```python
from build123d import *
from build123d.topology import SkipClean

# Parameters (mm, degrees)
EXTRUDE_1_DEPTH       = 200
MIRROR_2_COPY_1_DEPTH = 200
FILLET_1_R            = 2


with BuildPart() as part:
    # Sketch 1 → Extrude 1 (new, symmetric)
    with BuildSketch(Plane.XY):
        with BuildLine():
            Line((3, 14), (0, 14))
            Line((0, 14), (0, 12.5))
            ThreePointArc((0, 12.5), (1.767766953, 11.767766953), (2.5, 10))
            ThreePointArc((2.5, 10), (1.767766953, 8.232233047), (0, 7.5))
            Line((0, 7.5), (0, 6))
            Line((0, 6), (3, 6))
            Line((3, 6), (5.5, 3.5))
            Line((5.5, 3.5), (5.991970664, 3))
            Line((5.991970664, 3), (8, 3))
            Line((8, 3), (8, 0))
            Line((8, 0), (10, 0))
            Line((10, 0), (10, 5.641940268))
            ThreePointArc((10, 5.641940268), (9.646446609, 5.788386877), (9.5, 6.141940268))
            Line((9.5, 6.141940268), (8, 6.141940268))
            Line((8, 6.141940268), (8, 4.641940268))
            Line((8, 4.641940268), (6.5, 4.641940268))
            Line((6.5, 4.641940268), (4.740462433, 6.401477835))
            Line((4.740462433, 6.401477835), (4.740462433, 13.598522165))
            Line((4.740462433, 13.598522165), (6.5, 15.358059732))
            Line((6.5, 15.358059732), (8, 15.358059732))
            Line((8, 15.358059732), (8, 13.858059732))
            Line((8, 13.858059732), (9.5, 13.858059732))
            ThreePointArc((9.5, 13.858059732), (9.646446609, 14.211613123), (10, 14.358059732))
            Line((10, 14.358059732), (10, 20))
            Line((10, 20), (4.5, 20))
            ThreePointArc((4.5, 20), (4.353553391, 19.646446609), (4, 19.5))
            Line((4, 19.5), (4, 18))
            Line((4, 18), (5.5, 18))
            Line((5.5, 18), (5.5, 16.5))
            Line((5.5, 16.5), (3, 14))
        make_face()
    extrude_1 = extrude(amount=EXTRUDE_1_DEPTH, both=True)

    # Mirror 1: Extrude 1 across plane
    with SkipClean():  # the faces are left unmerged after this step: merging them gives an invalid solid
        add(extrude_1.mirror(Plane(origin=(0, 0, 0), x_dir=(0, 0, 1), z_dir=(1, 0, 0))))

    # Mirror 2: Extrude 1 across plane
    with SkipClean():  # the faces are left unmerged after this step: merging them gives an invalid solid
        add(extrude_1.mirror(Plane.ZX))

    # Mirror 2 copy 1 sketch → Mirror 2 copy 1 (add, symmetric)
    with SkipClean():  # the faces are left unmerged after this step: merging them gives an invalid solid
        with BuildSketch(Plane(origin=(0, 0, 0), x_dir=(-1, 0, 0), z_dir=(0, 0, 1))):
            with BuildLine():
                Line((3, 14), (0, 14))
                Line((0, 14), (0, 12.5))
                ThreePointArc((0, 12.5), (1.767766953, 11.767766953), (2.5, 10))
                ThreePointArc((2.5, 10), (1.767766953, 8.232233047), (0, 7.5))
                Line((0, 7.5), (0, 6))
                Line((0, 6), (3, 6))
                Line((3, 6), (5.5, 3.5))
                Line((5.5, 3.5), (5.991970664, 3))
                Line((5.991970664, 3), (8, 3))
                Line((8, 3), (8, 0))
                Line((8, 0), (10, 0))
                Line((10, 0), (10, 5.641940268))
                ThreePointArc((10, 5.641940268), (9.646446609, 5.788386877), (9.5, 6.141940268))
                Line((9.5, 6.141940268), (8, 6.141940268))
                Line((8, 6.141940268), (8, 4.641940268))
                Line((8, 4.641940268), (6.5, 4.641940268))
                Line((6.5, 4.641940268), (4.740462433, 6.401477835))
                Line((4.740462433, 6.401477835), (4.740462433, 13.598522165))
                Line((4.740462433, 13.598522165), (6.5, 15.358059732))
                Line((6.5, 15.358059732), (8, 15.358059732))
                Line((8, 15.358059732), (8, 13.858059732))
                Line((8, 13.858059732), (9.5, 13.858059732))
                ThreePointArc((9.5, 13.858059732), (9.646446609, 14.211613123), (10, 14.358059732))
                Line((10, 14.358059732), (10, 20))
                Line((10, 20), (4.5, 20))
                ThreePointArc((4.5, 20), (4.353553391, 19.646446609), (4, 19.5))
                Line((4, 19.5), (4, 18))
                Line((4, 18), (5.5, 18))
                Line((5.5, 18), (5.5, 16.5))
                Line((5.5, 16.5), (3, 14))
            make_face()
        extrude(amount=MIRROR_2_COPY_1_DEPTH, both=True)

    # Fillet 1
    fillet_1_edges = [part.edges().sort_by_distance(p)[0] for p in [
        (-10, 20, 0),
        (-10, -20, 0),
        (10, -20, 0),
        (10, 20, 0),
    ]]
    fillet(fillet_1_edges, radius=FILLET_1_R)


solid = part.part
```
Build history of the part. All positions in model axes, mm. A direction names the side the tool comes from. Round coordinates to 2 decimals unless told otherwise and drop trailing zeros. Put each result on its own line as item: value.
Item 1: Flat gauge pins, fed straight in: P1, Ø1.5, axis at x = 5, y = -1.5, coming from the +Z side; P2, Ø6, axis at y = 9.5, z = -58.5, coming from the -X side; P3, Ø1.5, axis at y = -10.5, z = 58, coming from the +X side; P4, Ø0.8, axis at x = 8.5, z = -40.5, coming from the -Y side. Where does each tip first touch, or does it go through?
Here are the results:
P1: passes through
P2: stops at x = -4.74
P3: stops at x = 4.74
P4: stops at y = -20
Item 2: Wall check: probe 1 along Y at (x, z) = (-8.5, 37); probe 2 along Y at (x, z) = (-7.75, -19); probe 3 along X at (y, z) = (1.5, 107). Give the ranges that are in metal, low to high. Write a range as from..to.
Here are the results:
probe 1: y = -19.94..-13.86, -6.14..6.14, 13.86..19.94
probe 2: y = -20..-15.36, -4.64..-3, 3..4.64, 15.36..20
probe 3: x = -10..-8, 8..10
Item 3: Tool access for faces 3 (the face through (4.74, -10, 3)), 4 (the face through (-4.74, 10, 3)), 5 (the face through (5, -5, -200)): list every direction of +Z, -Z, +X, -X, +Y, -Y with a clear straight run to the whole face (end or side of a thin tool).
Here are the results:
face 3: +Z, -Z, +X
face 4: +Z, -Z, -X
face 5: -Z, +X, -X, +Y, -Y
Item 4: Two-plate mould, pull along Y, no slides. Class faces 1 (the face through (5, -5, 200)), 2 (the face through (-4.74, -10, 3)): pulls with the +Y half, pulls with the -Y half, needs draft (parallel to the pull), parting line crosses it, or undercut.
Here are the results:
face 1: needs draft
face 2: undercut
Item 5: Slice it at A-A, the plane z = 54. Count the separate pieces of the cut face and the enclosed holes in it, plus the area to 3 significant figures.
Here are the results:
separate pieces: 1
enclosed holes: 3
area: 308 mm^2
